```python
from build123d import *

# Parameters (mm, degrees)
SKETCH1_W                       = 12.7
SKETCH1_H                       = 75
BOSS_EXTRUDE1_DEPTH             = 6.35
TAP_DRILL_FOR_M4X0_7_TAP1_D     = 3.3
SKETCH7_R                       = 4.75
CUT_EXTRUDE1_DEPTH              = 41.098160806
TAP_DRILL_FOR_M5X0_8_TAP1_D     = 4.2
TAP_DRILL_FOR_M5X0_8_TAP1_DEPTH = 15
TAP_DRILL_FOR_M5X0_8_TAP1_TIP   = 1.2618073


with BuildPart() as part:
    # Sketch1 → Boss-Extrude1 (new, symmetric)
    with BuildSketch(Plane(origin=(0, 0, 0), x_dir=(1, 0, 0), z_dir=(0, 1, 0))):
        Rectangle(SKETCH1_W, SKETCH1_H)
    extrude(amount=BOSS_EXTRUDE1_DEPTH, both=True)

    # Tap Drill for M4x0.7 Tap1 (through all)
    with Locations(Plane(origin=(0, 6.35, 0), x_dir=(1, 0, 0), z_dir=(0, 1, 0))):
        with Locations((0, -32.5), (0, -17.5)):
            Hole(TAP_DRILL_FOR_M4X0_7_TAP1_D / 2)

    # Sketch7 → Cut-Extrude1 (cut, through all)
    with BuildSketch(Plane.ZY.offset(6.35)):
        with Locations((-3.75, 0)):
            Circle(SKETCH7_R)
        with Locations((3.75, 0)):
            Circle(SKETCH7_R)
    extrude(amount=-CUT_EXTRUDE1_DEPTH, mode=Mode.SUBTRACT)

    # Tap Drill for M5x0.8 Tap1
    with Locations(Plane(origin=(0, 6.35, 0), x_dir=(1, 0, 0), z_dir=(0, 1, 0))):
        with Locations((0, 17.5), (0, 32.5)):
            Hole(TAP_DRILL_FOR_M5X0_8_TAP1_D / 2, depth=TAP_DRILL_FOR_M5X0_8_TAP1_DEPTH)
            with Locations((0, 0, -(TAP_DRILL_FOR_M5X0_8_TAP1_DEPTH + TAP_DRILL_FOR_M5X0_8_TAP1_TIP / 2))):  # 118° drill point
                Cone(0, TAP_DRILL_FOR_M5X0_8_TAP1_D / 2, TAP_DRILL_FOR_M5X0_8_TAP1_TIP, mode=Mode.SUBTRACT)


solid = part.part
```
For this review, take the finished solid that the model builds, in its own axes (mm). Coordinates: 2 decimals unless noted, no trailing zeros. Loops run counter-clockwise (first coordinate to the right, second up) from the corner with the lowest first, then second, coordinate; pieces in that order, holes last. Notation, with made-up numbers: (42.25, 58) - (94.25, 58) arc R19 cw to (94.25, 64) - close; hole circle Ø3 at (34.25, 78.5). An arc over 180 degrees is marked (long way). Use one line per item in the form item = value. Start each with the question number.
1) Take a section at B-B (y = 0). State the section outline as (x, z) points, plus the area to 3 significant figures.
2) Take a section at A-A (z = -3.75). State the section outline as (x, y) points.
3) To check wall thickness, follow probe 1 along Y at (x, z) = (-4, -3.75); probe 2 along Z at (x, y) = (6.25, -0.25); probe 3 along X at (y, z) = (-1, 32.5). State the ranges of each line that lie inside material, in increasing order. Write a range as from..to.
4) Take a section at D-D (y = 4). State the section outline as (x, z) points.
5) Take a section at C-C (x = 0). State the section outline as (y, z) points.
6) Draft analysis for pull direction Y (two halves, no side actions). For faces 1 (the face through (0, 6.35, -1)), 2 (the face through (6.35, 4.3, 0.5)), 3 (the face through (-0.089, 0.165, -8.497)), state which applies: released by +Y, released by -Y, zero draft, split by the parting line, or undercut.
From the geometry:
q1.outline = (-6.35, -37.5) - (6.35, -37.5) - (6.35, -8.5) - (-6.35, -8.5) - close; (-6.35, 8.5) - (6.35, 8.5) - (6.35, 37.5) - (-6.35, 37.5) - close; hole circle Ø4.2 at (0, -32.5); hole circle Ø4.2 at (0, -17.5); hole circle Ø3.3 at (0, 17.5); hole circle Ø3.3 at (0, 32.5)
q1.area = 692 mm2
q2.outline = (-6.35, -6.35) - (6.35, -6.35) - (6.35, -4.75) - (-6.35, -4.75) - close; (-6.35, 4.75) - (6.35, 4.75) - (6.35, 6.35) - (-6.35, 6.35) - close
q3.probe_1 = -6.35..-4.75, 4.75..6.35
q3.probe_2 = -37.5..-8.49, 8.49..37.5
q3.probe_3 = -6.35..-1.65, 1.65..6.35
q4.outline = (-6.35, -37.5) - (6.35, -37.5) - (6.35, -6.31) - (-6.35, -6.31) - close; (-6.35, -1.19) - (6.35, -1.19) - (6.35, 1.19) - (-6.35, 1.19) - close; (-6.35, 6.31) - (6.35, 6.31) - (6.35, 37.5) - (-6.35, 37.5) - close; hole circle Ø4.2 at (0, -32.5); hole circle Ø4.2 at (0, -17.5); hole circle Ø3.3 at (0, 17.5); hole circle Ø3.3 at (0, 32.5)
q5.outline = (-6.35, -37.5) - (6.35, -37.5) - (6.35, -34.6) - (-6.35, -34.6) - close; (-6.35, -30.4) - (6.35, -30.4) - (6.35, -19.6) - (-6.35, -19.6) - close; (-6.35, -15.4) - (6.35, -15.4) - (6.35, 15.85) - (-6.35, 15.85) - close; (-6.35, 19.15) - (6.35, 19.15) - (6.35, 30.85) - (-6.35, 30.85) - close; (-6.35, 34.15) - (6.35, 34.15) - (6.35, 37.5) - (-6.35, 37.5) - close; hole (-2.92, 0) arc R4.75 ccw (long way) to (2.92, 0) arc R4.75 ccw (long way) to start
q6.face_1 = released by +Y
q6.face_2 = zero draft
q6.face_3 = undercut
